```python
from build123d import *

# Parameters (mm, degrees)
Y_KSEKLIK_EKSTR_ZYON1_DEPTH      = 7.5
Y_KSEKLIK_EKSTR_ZYON1_DEPTH_BACK = 7.5
KES_EKSTR_ZYON1_DEPTH            = 9
IZIM3_R                          = 1.75
KES_EKSTR_ZYON2_DEPTH            = 7.5
IZIM4_W                          = 0.2
IZIM4_H                          = 4
KES_EKSTR_ZYON3_DEPTH            = 0.2


with BuildPart() as part:
    # izim1 → Y_kseklik-Ekstr_zyon1 (new body, two sides)
    with BuildSketch(Plane(origin=(0, 0, 0), x_dir=(0, 0, -1), z_dir=(1, 0, 0))) as y_kseklik_ekstr_zyon1_sk:
        Polygon((-1.856187291, 5), (3.143812709, 5), (4, 1), (4, -5.5), (-4, -5.5), (-4, 1), align=None)
    extrude(amount=Y_KSEKLIK_EKSTR_ZYON1_DEPTH)
    extrude(y_kseklik_ekstr_zyon1_sk.sketch, amount=-Y_KSEKLIK_EKSTR_ZYON1_DEPTH_BACK)

    # izim2 → Kes-Ekstr_zyon1 (cut, through all)
    with BuildSketch(Plane(origin=(0, 0, -4), x_dir=(-1, 0, 0), z_dir=(0, 0, -1))):
        Polygon((-0.5, -4.5), (-0.5, -5.5), (0.5, -5.5), (0.5, -4.5), (2, -4.5), (2, 0.5), (-2, 0.5), (-2, -4.5), align=None)
        Polygon((3, 0.5), (3, -4.5), (4.5, -4.5), (4.5, -5.5), (5.5, -5.5), (5.5, -4.5), (7, -4.5), (7, 0.5), align=None)
        Polygon((-7, 0.5), (-7, -4.5), (-5.5, -4.5), (-5.5, -5.5), (-4.5, -5.5), (-4.5, -4.5), (-3, -4.5), (-3, 0.5), align=None)
    extrude(amount=-KES_EKSTR_ZYON1_DEPTH, mode=Mode.SUBTRACT)

    # izim3 → Kes-Ekstr_zyon2 (cut)
    with BuildSketch(Plane(origin=(0, 5, 0), x_dir=(1, 0, 0), z_dir=(0, 1, 0))):
        with Locations((0, 0.643812709)):
            Circle(IZIM3_R)
        with Locations((-5, 0.643812709)):
            Circle(IZIM3_R)
        with Locations((5, 0.643812709)):
            Circle(IZIM3_R)
    extrude(amount=-KES_EKSTR_ZYON2_DEPTH, mode=Mode.SUBTRACT)

    # izim4 → Kes-Ekstr_zyon3 (cut)
    with BuildSketch(Plane(origin=(0, 5, 0), x_dir=(1, 0, 0), z_dir=(0, 1, 0))):
        with Locations((-2.5, 0.643812709)):
            Rectangle(IZIM4_W, IZIM4_H)
        with Locations((2.5, 0.643812709)):
            Rectangle(IZIM4_W, IZIM4_H)
    extrude(amount=-KES_EKSTR_ZYON3_DEPTH, mode=Mode.SUBTRACT)


solid = part.part
```
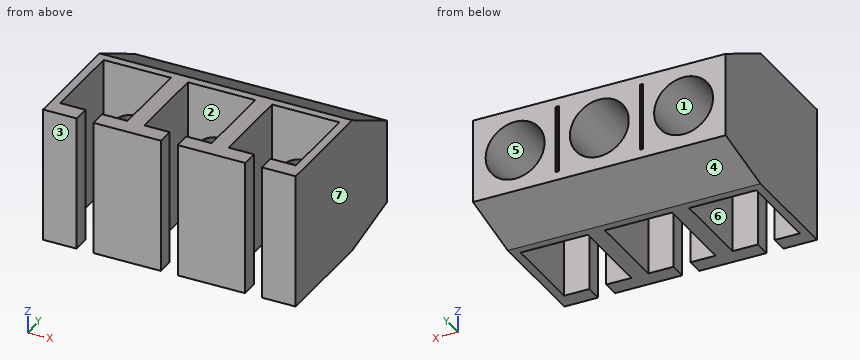
Model file for the job. Use its own axes, mm. Face numbers are marked on the shaded views. A direction names the side the tool comes from. Coordinates: 2 decimals unless noted, no trailing zeros. Order: outer loops, then holes, each group sorted by start corner. A loop starts at its lowest first (then second) coordinate and runs counter-clockwise, first axis right, second up. Notation, with made-up numbers: (72, -5.5) -> (110, -5.5) arc R19 cw to (110, 11.5) -> close; hole circle Ø5 at (3.25, 40). An arc over 180 degrees is marked (long way). Answer as a JSON object with one key per item and string values. Group by question number.
1) Cut at C-C, the plane x = -3.5. Write the cut outline in (y, z).
2) Drill centre lines: L1, parallel to X at y = -3, z = 1.25; L2, parallel to X at y = -4.75, z = 0.75; L3, parallel to Y at x = 6, z = 1.75. Where is each one in solid material? Low to high.
3) Pull direction X, two halves, no side cores. Call the marked faces 4, 5, 6 and 7: +X half, -X half, draft (parallel to the pull), parting line (faces both ways), or undercut.
4) Cut at B-B, the plane y = -2.75. Write the cut outline in (x, z), then the cut area to 3 significant figures.
5) Flat gauge pins, fed straight in: pin 1 (1.2 mm diameter, centred on x = 4, z = -1, fed in from +Y); pin 2 (1 mm diameter, centred on x = -0.5, y = 3, fed in from -Z). Where does each tip first touch, or does it go through?
6) Cut at A-A, the plane x = 5. Write the cut outline in (y, z), then the cut area to 4 significant figures.
7) Which spindle directions (+Z, -Z, +X, -X, +Y, -Y) get a long thin tool onto all of the face, cutting with end or side? Do the marked faces 1, 2 and 3. Say none if no direction does.
8) Cut at D-D, the plane z = 2.5. Write the cut outline in (x, y), then the cut area to 3 significant figures.
Check values:
{
 "1": {"outline": "(-5.5, -4) -> (-4.5, -4) -> (-4.5, 4) -> (-5.5, 4) -> close; (0.5, -4) -> (1, -4) -> (5, -3.14) -> (5, -1.55) -> (0.5, -1.55) -> close; (0.5, 0.26) -> (5, 0.26) -> (5, 1.86) -> (1, 4) -> (0.5, 4) -> close"},
 "2": {"L1": "x = -7.5 to -7, -3 to -2, 2 to 3, 7 to 7.5", "L2": "x = -7.5 to -5.5, -4.5 to -0.5, 0.5 to 4.5, 5.5 to 7.5", "L3": "y = -5.5 to -4.5, 0.5 to 5"},
 "3": {"face 4": "draft", "face 5": "undercut", "face 6": "undercut", "face 7": "+X half"},
 "4": {"outline": "(-7.5, -4) -> (-7, -4) -> (-7, 4) -> (-7.5, 4) -> close; (-3, -4) -> (-2, -4) -> (-2, 4) -> (-3, 4) -> close; (2, -4) -> (3, -4) -> (3, 4) -> (2, 4) -> close; (7, -4) -> (7.5, -4) -> (7.5, 4) -> (7, 4) -> close", "area": "24.0 mm²"},
 "5": {"pin 1": "stops at y = -4.5", "pin 2": "stops at z = -3.68"},
 "6": {"outline": "(0.5, -4) -> (1, -4) -> (5, -3.14) -> (5, -2.39) -> (0.5, -2.39) -> close; (0.5, 1.11) -> (5, 1.11) -> (5, 1.86) -> (1, 4) -> (0.5, 4) -> close", "area": "14.25 mm²"},
 "7": {"face 1": "+Y", "face 2": "+Z, -Z", "face 3": "+Z, -Z, +X, -X, -Y"},
 "8": {"outline": "(-7.5, -5.5) -> (-5.5, -5.5) -> (-5.5, -4.5) -> (-7, -4.5) -> (-7, 0.5) -> (-3, 0.5) -> (-3, -4.5) -> (-4.5, -4.5) -> (-4.5, -5.5) -> (-0.5, -5.5) -> (-0.5, -4.5) -> (-2, -4.5) -> (-2, 0.5) -> (2, 0.5) -> (2, -4.5) -> (0.5, -4.5) -> (0.5, -5.5) -> (4.5, -5.5) -> (4.5, -4.5) -> (3, -4.5) -> (3, 0.5) -> (7, 0.5) -> (7, -4.5) -> (5.5, -4.5) -> (5.5, -5.5) -> (7.5, -5.5) -> (7.5, 3.8) -> (-7.5, 3.8) -> close", "area": "76.5 mm²"}
}
